```python
from build123d import *

# Parameters (mm, degrees)
F0_W     = 5.97
F0_H     = 2.5
F0_W_2   = 6.31
F1_DEPTH = 10
F0_W_3   = 6.45
F0_H_2   = 2.33
F3_R     = 2.19
F3_R_2   = 2.195
F4_DEPTH = 2.5
F5_R     = 2.19
F6_DEPTH = 2.5
F7_R     = 1.5
F8_DEPTH = 3


with BuildPart() as f1:
    # F0 (on Front) → F1 (new body, symmetric)
    with BuildSketch(Plane.XZ):
        Polygon((-6.45, 9.35), (-9.66, 9.35), (-9.66, 2.5), (-9.66, 0), (-9.66, -26.67), (30.32, -26.67), (30.32, 0), (30.32, 2.5), (30.32, 9.35), (6.45, 9.35), (0, 9.35), align=None)
        with Locations((33.305, 1.25)):
            Rectangle(F0_W, F0_H)
        with Locations((-12.815, 1.25)):
            Rectangle(F0_W_2, F0_H)
    extrude(amount=F1_DEPTH, both=True)

    # F0 (on Front) → F2 (revolve)
    with BuildSketch(Plane.XZ):
        with Locations((3.225, 10.515)):
            Rectangle(F0_W_3, F0_H_2)
    revolve(axis=Axis((0, 0, -16.804387), (0, 0, -1)))

    # F3 (on face) → F4 (cut, through all)
    with BuildSketch(Plane(origin=(0, 0, 0), x_dir=(1, 0, 0), z_dir=(0, 0, -1))):
        with Locations((-13.47, 5.085)):
            Circle(F3_R)
        with Locations((-13.47, -5.085)):
            Circle(F3_R_2)
    extrude(amount=-F4_DEPTH, mode=Mode.SUBTRACT)

    # F5 (on face) → F6 (cut, through all)
    with BuildSketch(Plane(origin=(0, 0, 0), x_dir=(1, 0, 0), z_dir=(0, 0, -1))):
        with Locations((33.79, 5.085)):
            Circle(F5_R)
        with Locations((33.79, -5.085)):
            Circle(F5_R)
    extrude(amount=-F6_DEPTH, mode=Mode.SUBTRACT)

    # F7 (on face) → F8 (join)
    with BuildSketch(Plane.XY.offset(11.68)):
        Circle(F7_R)
    extrude(amount=F8_DEPTH)


solid = f1.part
```
CAD build for the part. Positions are in the model's coordinates, mm. A direction names the side the tool comes from. Give positions to 0.01 mm unless a question says otherwise; leave off trailing zeros. Write each loop counter-clockwise with the first axis right and the second up, starting at its lowest first coordinate (ties: lowest second). Pieces come first, ordered by that corner, then holes. Notation, with made-up numbers: (-0.5, 56) -> (46.5, 56) arc R35 ccw to (46.5, 92) -> close; hole circle Ø10 at (61.5, 36). An arc over 180 degrees is marked (long way). Write each question's results on one line, items separated by ' | '.
1. Cut at B-B, the plane y = 0. Write the cut outline in (x, z), then the cut area to 3 significant figures.
Geometry check:
outline: (-15.97, 0) -> (-9.66, 0) -> (-9.66, -26.67) -> (30.32, -26.67) -> (30.32, 0) -> (36.29, 0) -> (36.29, 2.5) -> (30.32, 2.5) -> (30.32, 9.35) -> (6.45, 9.35) -> (6.45, 11.68) -> (1.5, 11.68) -> (1.5, 14.68) -> (-1.5, 14.68) -> (-1.5, 11.68) -> (-6.45, 11.68) -> (-6.45, 9.35) -> (-9.66, 9.35) -> (-9.66, 2.5) -> (-15.97, 2.5) -> close | area: 1,510 mm²
2. Cut at C-C, the plane x = 0. Write the cut outline in (y, z), then the cut area to 3 significant figures.
Geometry check:
outline: (-10, -26.67) -> (10, -26.67) -> (10, 9.35) -> (6.45, 9.35) -> (6.45, 11.68) -> (1.5, 11.68) -> (1.5, 14.68) -> (-1.5, 14.68) -> (-1.5, 11.68) -> (-6.45, 11.68) -> (-6.45, 9.35) -> (-10, 9.35) -> close | area: 759 mm²
3. Which spindle directions (+Z, -Z, +X, -X, +Y, -Y) get a long thin tool onto all of the face, cutting with end or side? Do faces 1 (the flat face through (33, 0, 2.5)), 2 (the flat face through (-9.66, 0, 6)), 3 (the cylindrical face through (-1.398, 6.297, 10.531)), 4 (the flat face through (30.32, 0, -14)). Say none if no direction does.
Geometry check:
face 1: +Z, +X, +Y, -Y | face 2: +Z, -X, +Y, -Y | face 3: +Z | face 4: -Z, +X, +Y, -Y
4. Wall check: probe 1 along Y at (x, z) = (-13.47, 1.8) (3 decimals); probe 2 along X at (y, z) = (-4.75, 1.5); probe 3 along Y at (x, z) = (-13, 1). Give the ranges that are in metal, low to high. Write a range as [from, to].
Geometry check:
probe 1: [-10, -7.275], [-2.895, 2.89], [7.28, 10] | probe 2: [-15.97, -15.63], [-11.31, 31.63], [35.95, 36.29] | probe 3: [-10, -7.22], [-2.95, 2.94], [7.23, 10]
5. Cut at D-D, the plane y = -4.25. Write the cut outline in (x, z), then the cut area to 3 significant figures.
Geometry check:
outline: (-15.97, 0) -> (-15.49, 0) -> (-15.49, 2.5) -> (-15.97, 2.5) -> close; (-11.45, 0) -> (-9.66, 0) -> (-9.66, -26.67) -> (30.32, -26.67) -> (30.32, 0) -> (31.77, 0) -> (31.77, 2.5) -> (30.32, 2.5) -> (30.32, 9.35) -> (4.85, 9.35) -> (4.85, 11.68) -> (-4.85, 11.68) -> (-4.85, 9.35) -> (-9.66, 9.35) -> (-9.66, 2.5) -> (-11.45, 2.5) -> close; (35.81, 0) -> (36.29, 0) -> (36.29, 2.5) -> (35.81, 2.5) -> close | area: 1,470 mm²
6. Cut at A-A, the plane x = 33.79. Write the cut outline in (y, z) (3 decimals).
Geometry check:
outline: (-10, 0) -> (-7.275, 0) -> (-7.275, 2.5) -> (-10, 2.5) -> close; (-2.895, 0) -> (2.895, 0) -> (2.895, 2.5) -> (-2.895, 2.5) -> close; (7.275, 0) -> (10, 0) -> (10, 2.5) -> (7.275, 2.5) -> close
7. Drop flat-ended pins along their axis: P1, Ø4, axis at x = 33.79, y = 5.085, coming from the -Z side; P2, Ø6, axis at x = 5, y = 3.5, coming from the +Z side; P3, Ø4, axis at x = -8.5, y = -5, coming from the +Z side; P4, Ø1, axis at y = 1.5, z = -22, coming from the -X side. Give the stop position or say it passes through.
Geometry check:
P1: through | P2: z = 11.68 | P3: z = 9.35 | P4: x = -9.66
8. Two-plate mould, pull along Y, no slides. Class faces 5 (the cylindrical face through (-1.5, 0.07, 13.16)), 6 (the cylindrical face through (-15.658, -5.181, 1.232)), 7 (the cylindrical face through (31.6, 5, 1.2)), 8 (the flat face through (-15.97, 0, 1)): pulls with the +Y half, pulls with the -Y half, needs draft (parallel to the pull), parting line crosses it, or undercut.
Geometry check:
face 5: parting line crosses it | face 6: undercut | face 7: undercut | face 8: needs draft
